from build123d import *

# Parameters (mm, degrees)
F0_W     = 2.5
F0_H     = 4
F0_R     = 2.3114
F1_DEPTH = 3.175


with BuildPart() as f1:
    # F0 (on Top) → F1 (new body)
    with BuildSketch(Plane.XY):
        with BuildLine():
            Line((-451.5609132883, 3.4527331373), (-420.9521720122, 3.4527331373))
            Line((-420.9521720122, 3.4527331373), (-359.0199119076, 91.1230753634))
            Line((-359.0199119076, 91.1230753634), (-379.4389155629, 105.5475091382))
            Line((-379.4389155629, 105.5475091382), (-386.6511324503, 95.3380073106))
            Line((-386.6511324503, 95.3380073106), (-378.3294900246, 89.4594158723))
            ThreePointArc((-378.3294900246, 89.4594158723), (-375.7419979554, 90.3287620732), (-374.1302306227, 88.1257904232))
            ThreePointArc((-374.1302306227, 88.1257904232), (-375.3786094336, 86.0733392273), (-377.7752560717, 86.2379310212))
            Line((-377.7752560717, 86.2379310212), (-424.151080008, 20.5890373971))
            ThreePointArc((-424.151080008, 20.5890373971), (-423.4322542612, 19.7641991843), (-423.1733054571, 18.7011779952))
            ThreePointArc((-423.1733054571, 18.7011779952), (-426.1843381244, 16.4982063451), (-427.3725648591, 20.0348034442))
            Line((-427.3725648591, 20.0348034442), (-435.6942072848, 25.9133948826))
            Line((-435.6942072848, 25.9133948826), (-451.5609132883, 3.4527331373))
        make_face()
        Polygon((-359.0199119076, 91.1230753634), (-420.9521720122, 3.4527331373), (-227, 3.4527331373), (-227, 56.2263665687), (-227, 61.5263665687), (-232, 61.5263665687), (-232, 65.5263665687), (-227, 65.5263665687), (-227, 77.2140920162), (-227, 109), (-277, 109), (-377, 109), (-379.4389155629, 105.5475091382), align=None)
        with Locations((-263.75, 56.2263665687)):
            Rectangle(F0_W, F0_H, mode=Mode.SUBTRACT)
        with BuildLine():
            ThreePointArc((-274.6886, 96.5), (-278.634406614, 94.865593386), (-277, 98.8114))
            ThreePointArc((-277, 98.8114), (-275.365593386, 98.134406614), (-274.6886, 96.5))
        make_face(mode=Mode.SUBTRACT)
        Polygon((-227, 56.2263665687), (-227, 3.4527331373), (-2.4390867117, 3.4527331373), (-77, 109), (-177, 109), (-227, 109), (-227, 77.2140920162), (-227, 65.5263665687), (-222, 65.5263665687), (-222, 61.5263665687), (-227, 61.5263665687), align=None)
        with Locations((-28.5152945429, 18.7011779952)):
            Circle(F0_R, mode=Mode.SUBTRACT)
        Polygon((-191.5, 54.2263665687), (-191.5, 56.2263665687), (-191.5, 58.2263665687), (-189, 58.2263665687), (-189, 54.2263665687), align=None, mode=Mode.SUBTRACT)
        with Locations((-77.5583693773, 88.1257904232)):
            Circle(F0_R, mode=Mode.SUBTRACT)
        with BuildLine():
            ThreePointArc((-174.6886, 96.5), (-177, 94.1886), (-179.3114, 96.5))
            ThreePointArc((-179.3114, 96.5), (-178.634406614, 98.134406614), (-177, 98.8114))
            ThreePointArc((-177, 98.8114), (-175.365593386, 98.134406614), (-174.6886, 96.5))
        make_face(mode=Mode.SUBTRACT)
        with BuildLine():
            Line((-415.5, 54.5), (-435.6942072848, 25.9133948826))
            Line((-435.6942072848, 25.9133948826), (-427.3725648591, 20.0348034442))
            ThreePointArc((-427.3725648591, 20.0348034442), (-425.8766080436, 20.9791117788), (-424.151080008, 20.5890373971))
            Line((-424.151080008, 20.5890373971), (-377.7752560717, 86.2379310212))
            ThreePointArc((-377.7752560717, 86.2379310212), (-378.7195644063, 87.7338878367), (-378.3294900246, 89.4594158723))
            Line((-378.3294900246, 89.4594158723), (-386.6511324503, 95.3380073106))
            Line((-386.6511324503, 95.3380073106), (-415.5, 54.5))
        make_face()
    extrude(amount=F1_DEPTH)


solid = f1.part
Verification items for the finished model (mm, model axes). Give positions to 0.01 mm unless a question says otherwise; leave off trailing zeros. Write each loop counter-clockwise with the first axis right and the second up, starting at its lowest first coordinate (ties: lowest second). Pieces come first, ordered by that corner, then holes.
(1) Material ranges on line 1 (X direction, y = 63, z = 3); line 2 (X direction, y = 55, z = 1.45); line 3 (X direction, y = 97, z = 1.3), recorded low to high.
(2) Gauge pin test, flat ends, axial feed: pin 1 (1.6 mm diameter, centred on y = 64, z = 1, fed in from -X); pin 2 (1.6 mm diameter, centred on y = 56, z = 2.5, fed in from +X); pin 3 (1.6 mm diameter, centred on y = 55.5, z = 2, fed in from +X). Record the tip position at first contact, or that the pin passes through.
(3) Cross-section at A-A (z = 1.75). State how many separate pieces and enclosed holes the cut face has, plus the area to 3 significant figures.
(4) Cross-section at C-C (x = -37.5). Enter the section's corners in (y, z) (3 decimals).
(5) Cross-section at B-B (x = -409). Enter the section's corners in (y, z) (3 decimals).
Worked out:
1. line 1: x = -409.5 to -232, -222 to -44.5
1. line 2: x = -415.15 to -265, -262.5 to -191.5, -189 to -38.85
1. line 3: x = -385.48 to -279.26, -274.74 to -179.26, -174.74 to -68.52
2. pin 1: stops at x = -409.35
2. pin 2: stops at x = -38.99
2. pin 3: stops at x = -38.64
3. separate pieces: 1
3. enclosed holes: 9
3. area: 39,400 mm2
4. outline: (3.453, 0) - (53.084, 0) - (53.084, 3.175) - (3.453, 3.175) - close
5. outline: (3.453, 0) - (63.701, 0) - (63.701, 3.175) - (3.453, 3.175) - close
